The figure shows three views and two pictorial views of one solid part (mm, origin at its lowest corner). Answer the questions. A direction names the side the tool comes from. Coordinates: 2 decimals unless noted, no trailing zeros. Loops run counter-clockwise (first coordinate to the right, second up) from the corner with the lowest first, then second, coordinate; pieces in that order, holes last. Notation, with made-up numbers: M 40,75.25 L 44,75.25 A5 ccw 44,82.25 Z; hole C -20.5,-20 d4. An arc over 180 degrees is marked long. Return JSON: item names as keys, results as strings. Group by question number.
1. Section C-C (z = 19) is taken. Write down the section's boundary in (x, y), then the cut area to 3 significant figures.
2. Section B-B (x = 60.5) is taken. Write down the section's boundary in (y, z).
3. Straight lines are drawn through the part: L1, parallel to X at y = 26, z = 24.5; L2, parallel to Z at x = 39.5, y = 93.5; L3, parallel to Y at x = 71, z = 14.5. For each, find the intervals that lie inside material, in ascending order. Write a range as from..to.
4. Section D-D (x = 19.5) is taken. Write down the section's boundary in (y, z).
5. Given P1, Ø6, axis at x = 49.5, y = 93, coming from the -Z side; P2, Ø2, axis at x = 10, z = 11, coming from the -Y side; P3, Ø0.6, axis at x = 85, y = 120.5, coming from the +Z side, each flat-ended and moving along its own axis, determine where each tip first touches the part or whether it passes through.
6. The mould has two halves that part along X. Classify the marked faces 4 and 5: pulls with the +X half, pulls with the -X half, needs draft (parallel to the pull), parting line crosses it, or undercut.
7. Which of the six approach directions +Z, -Z, +X, -X, +Y, -Y give full straight-line access (tool end or side, diameter ignored) to the marked faces 1, 2 and 3?
8. Section A-A (y = 100.5) is taken. Write down the section's boundary in (x, z).
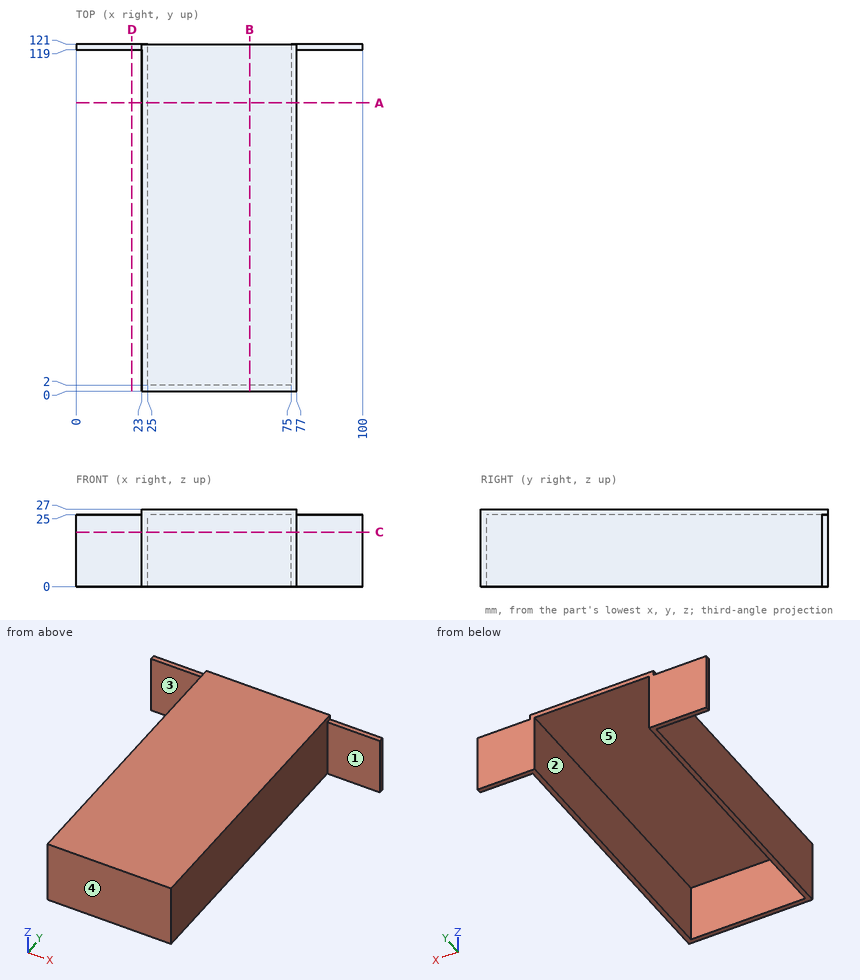
Worked out:
{
 "1": {"outline": "M 0,119 L 23,119 L 23,0 L 77,0 L 77,119 L 100,119 L 100,121 L 75,121 L 75,2 L 25,2 L 25,121 L 0,121 Z", "area": "676 mm^2"},
 "2": {"outline": "M 0,0 L 2,0 L 2,25 L 121,25 L 121,27 L 0,27 Z"},
 "3": {"L1": "23..25, 75..77", "L2": "25..27", "L3": "0..2"},
 "4": {"outline": "M 119,0 L 121,0 L 121,25 L 119,25 Z"},
 "5": {"P1": "z = 25", "P2": "y = 119", "P3": "z = 25"},
 "6": {"face 4": "needs draft", "face 5": "undercut"},
 "7": {"face 1": "+Z, -Z, +X, -Y", "face 2": "-Z, +Y", "face 3": "+Z, -Z, -X, -Y"},
 "8": {"outline": "M 23,0 L 25,0 L 25,25 L 75,25 L 75,0 L 77,0 L 77,27 L 23,27 Z"}
}
